Geometry: final body of the model. Coordinates: model frame, mm. Coordinates: 2 decimals unless noted, no trailing zeros. Order: outer loops, then holes, each group sorted by start corner. A loop starts at its lowest first (then second) coordinate and runs counter-clockwise, first axis right, second up. Notation, with made-up numbers: M -17.5,-12.75 L 33.5,-12.75 A29 ccw 33.5,19.25 Z; hole C 10,5.5 d8. An arc over 180 degrees is marked long. Use CSV: the item, a comma, the result in double quotes. Start each with the question number.
1. First-contact query: P1, Ø1.2, axis at x = -21, z = 1.5, coming from the -Y side; P2, Ø4, axis at x = -18, y = 28, coming from the +Z side. Flat tips, straight axial feed; report the tip coordinate or a pass-through.
2. Section query B-B on x = 13.5. Return the cut outline in (y, z).
3. Section query A-A on y = -24. Return the cut outline in (x, z).
4. Section query D-D on y = -6.5. Return the cut outline in (x, z), and give its area (3 significant figures).
5. Material intervals for line 1 (Y direction, x = 8, z = 2.6); line 2 (X direction, y = 11.5, z = 1.6); line 3 (Y direction, x = 18, z = 1), sorted ascending.
6. Section query C-C on z = 1. State how many separate pieces and enclosed holes the cut face has, and give its area (3 significant figures).
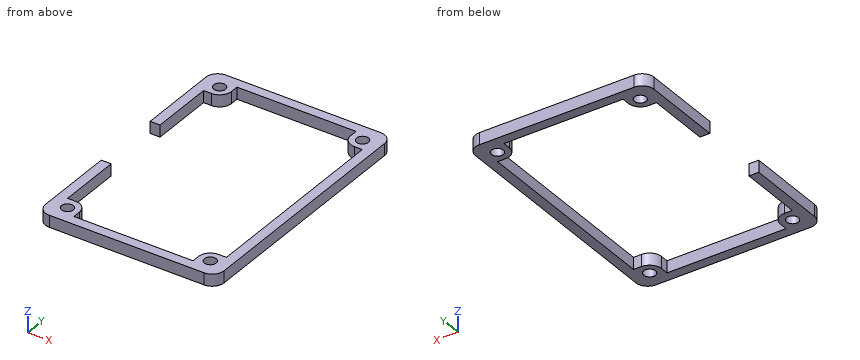
Autodesk Inventor part; units mm, degrees
ref_plane "YZ Plane" through (0, 0, 0) normal (1, 0, 0) x (0, 1, 0)
ref_plane "XZ Plane" through (0, 0, 0) normal (0, 1, 0) x (-1, 0, 0)
ref_plane "XY Plane" through (0, 0, 0) normal (0, 0, 1) x (1, 0, 0)
sketch "Эскиз1" plane through (0, 0, 0) normal (0, 0, 1) x (1, 0, 0)
  line L0 (19.5, 32.5) -> (-19.5, 32.5)
  line L1 (-22.5, 29.5) -> (-22.5, -29.5)
  line L2 (-19.5, -32.5) -> (19.5, -32.5)
  line L3 (22.5, -29.5) -> (22.5, 29.5)
  line L4 (22.5, 32.5) -> (-22.5, -32.5) construction
  line L5 (-22.5, 32.5) -> (22.5, -32.5) construction
  circle A0 centre (18, 28) radius 1.5
  circle A1 centre (18, -28) radius 1.5
  circle A2 centre (-18, -28) radius 1.5
  circle A3 centre (-18, 28) radius 1.5
  arc A4 (22.5, 29.5) -> (19.5, 32.5) centre (19.5, 29.5) ccw
  arc A5 (19.5, -32.5) -> (22.5, -29.5) centre (19.5, -29.5) ccw
  arc A6 (-22.5, -29.5) -> (-19.5, -32.5) centre (-19.5, -29.5) ccw
  arc A7 (-19.5, 32.5) -> (-22.5, 29.5) centre (-19.5, 29.5) ccw
  line L6 (20, -30) -> (20, 30)
  line L7 (20, 30) -> (-20, 30)
  line L8 (-20, 30) -> (-20, 9)
  line L9 (-20, -9) -> (-20, -30)
  line L10 (-20, -30) -> (20, -30)
  line L11 (20, -30) -> (15, -30)
  line L12 (15, -30) -> (15, -28)
  line L13 (18, -25) -> (20, -25)
  line L14 (20, -25) -> (20, -30)
  arc A8 (18, -25) -> (15, -28) centre (18, -28) ccw
  line L15 (20, 30) -> (15, 30)
  line L16 (15, 30) -> (15, 28)
  line L17 (18, 25) -> (20, 25)
  line L18 (20, 25) -> (20, 30)
  line L19 (-20, 30) -> (-15, 30)
  line L20 (-15, 30) -> (-15, 28)
  line L21 (-18, 25) -> (-20, 25)
  line L22 (-20, 25) -> (-20, 30)
  line L23 (-20, -30) -> (-15, -30)
  line L24 (-15, -30) -> (-15, -28)
  line L25 (-18, -25) -> (-20, -25)
  line L26 (-20, -25) -> (-20, -30)
  arc A9 (15, 28) -> (18, 25) centre (18, 28) ccw
  arc A10 (-18, 25) -> (-15, 28) centre (-18, 28) ccw
  arc A11 (-15, -28) -> (-18, -25) centre (-18, -28) ccw
  line L27 (-20, 9) -> (-22.5, 9)
  line L28 (-20, -9) -> (-22.5, -9)
  point P0 (0, 0)
  point P1 (15, -25)
  point P2 (15, 25)
  point P3 (-15, 25)
  point P4 (-15, -25)
  dimension "d0" = 45
  dimension "d1" = 65
  dimension "d2" = 3
  dimension "d3" = 5
  dimension "d4" = 5
  dimension "d5" = 3
  dimension "d6" = 5
  dimension "d7" = 5
  dimension "d8" = 5
  dimension "d9" = 5
  dimension "d10" = 5
  dimension "d11" = 3
extrude "Выдавливание1" add sketch "Эскиз1" along normal blind 3 contours A4 L3 A5 L2 A6 L1 L28 L9 L10 L6 L7 L8 L27 A7 L0 | L8 L7 L20 A10 L21 | L25 A11 L24 L10 L9 | L7 L6 L17 A9 L16 | L12 A8 L13 L6 L10
properties part number "level1_up"
Results list:
1,P1,"stops at y = -32.36"
1,P2,"stops at z = 3"
2,outline,"M -32.5,0 L -30,0 L -30,3 L -32.5,3 Z; M 30,0 L 32.5,0 L 32.5,3 L 30,3 Z"
3,outline,"M -22.5,0 L -20,0 L -20,3 L -22.5,3 Z; M 20,0 L 22.5,0 L 22.5,3 L 20,3 Z"
4,outline,"M 20,0 L 22.5,0 L 22.5,3 L 20,3 Z"
4,area,"7.50 mm²"
5,line 1,"y = -32.5 to -30, 30 to 32.5"
5,line 2,"x = -22.5 to -20, 20 to 22.5"
5,line 3,"y = -32.5 to -29.5, -26.5 to -25, 25 to 26.5, 29.5 to 32.5"
6,separate pieces,"1"
6,enclosed holes,"4"
6,area,"536 mm²"
